```python
from build123d import *

# Parameters (mm, degrees)
F0_W     = 72.736366
F0_H     = 121.693536
F1_DEPTH = 19.05
F2_W     = 63.592366
F2_H     = 56.449744
F2_R     = 3.556
F2_W_2   = 5.08
F2_H_2   = 1.524
F3_DEPTH = 1.27
F4_R     = 5.08


with BuildPart() as f1:
    # F0 (on Front) → F1 (new body)
    with BuildSketch(Plane.XZ):
        Rectangle(F0_W, F0_H)
    extrude(amount=F1_DEPTH)

    # F2 (on face) → F3 (join)
    with BuildSketch(Plane.XZ.offset(19.05)):
        with Locations((0, 27.541896)):
            Rectangle(F2_W, F2_H)
        Polygon((-14.500647, -17.314185), (-22.619766, -17.314185), (-22.619766, -26.204185), (-29.613647, -26.204185), (-29.613647, -34.332185), (-22.628647, -34.332185), (-22.628647, -43.222185), (-14.500647, -43.222185), (-14.500647, -34.332185), (-7.515647, -34.332185), (-7.515647, -26.204185), (-14.500647, -26.204185), align=None)
        with Locations((30.073691, -19.163234)):
            Circle(F2_R)
        with Locations((19.722743, -25.038093)):
            Circle(F2_R)
        with Locations((-5.588, -54.265258)):
            Rectangle(F2_W_2, F2_H_2)
        with Locations((5.588, -54.265258)):
            Rectangle(F2_W_2, F2_H_2)
    extrude(amount=F3_DEPTH)

    # F4
    f4_edges = [f1.edges().sort_by_distance(p)[0] for p in [
        (-36.368183, -9.525, 60.846768),
        (36.368183, -9.525, 60.846768),
        (36.368183, -9.525, -60.846768),
        (-36.368183, -9.525, -60.846768),
    ]]
    fillet(f4_edges, radius=F4_R)


solid = f1.part
```
The listing builds one solid part. Answer for the finished solid, in the listing's coordinates (mm). A direction names the side the tool comes from. Coordinates: 2 decimals unless noted, no trailing zeros. Loops run counter-clockwise (first coordinate to the right, second up) from the corner with the lowest first, then second, coordinate; pieces in that order, holes last. Notation, with made-up numbers: M 59,-3 L 113,-3 A34 cw 113,27 Z; hole C 6.25,-4.5 d1. An arc over 180 degrees is marked long. Answer as a JSON object with one key per item and string values. Group by question number.
Item 1: Section A-A (x = -25.5) is taken. Write down the section's boundary in (y, z), and give its area (3 significant figures).
Item 2: Section C-C (x = 11) is taken. Write down the section's boundary in (y, z).
Item 3: Which of the six approach directions +Z, -Z, +X, -X, +Y, -Y give full straight-line access (tool end or side, diameter ignored) to faces 1 (the face through (0, -9, 60.847)), 2 (the face through (33.359, -19.676, -20.525))?
Item 4: Section B-B (z = -8.5) is taken. Write down the section's boundary in (x, y).
Item 5: Consider L1, parallel to Y at x = -19.5, z = -47.5; L2, parallel to X at y = -19.5, z = -36; L3, parallel to Z at x = 33, y = -1. Determine where each line is inside the solid, lowest interval first.
Item 6: Section D-D (x = 21.5) is taken. Write down the section's boundary in (y, z), and give its area (3 significant figures).
Item 7: Determine the mould class of faces 3 (the face through (0, -9, -60.847)), 4 (the face through (-1, -19.05, -13)), 5 (the face through (23.008, -19.676, -26.4)), 6 (the face through (0, -20.32, 28)) for opening direction Z: +Z half, -Z half, draft (parallel to the pull), parting line (faces both ways), or undercut.
Item 8: Each of these flat-tipped pins is pushed along its axis until it touches: P1, Ø0.6, axis at y = -20, z = -21.5, coming from the +X side; P2, Ø0.6, axis at y = -19.5, z = -38, coming from the -X side; P3, Ø1.4, axis at x = -3, y = -20, coming from the +Z side. Where does it stop, or does it pass through?
Solved:
{
 "1": {"outline": "M -20.32,-34.33 L -19.05,-34.33 L -19.05,-60.85 L 0,-60.85 L 0,60.85 L -19.05,60.85 L -19.05,55.77 L -20.32,55.77 L -20.32,-0.68 L -19.05,-0.68 L -19.05,-26.2 L -20.32,-26.2 Z", "area": "2,400 mm2"},
 "2": {"outline": "M -20.32,-0.68 L -19.05,-0.68 L -19.05,-60.85 L 0,-60.85 L 0,60.85 L -19.05,60.85 L -19.05,55.77 L -20.32,55.77 Z"},
 "3": {"face 1": "+Z, +X, -X, +Y, -Y", "face 2": "-Y"},
 "4": {"outline": "M -36.37,-19.05 L 36.37,-19.05 L 36.37,0 L -36.37,0 Z"},
 "5": {"L1": "y = -19.05 to 0", "L2": "x = -22.63 to -14.5", "L3": "z = -60.55 to 60.55"},
 "6": {"outline": "M -20.32,-28.12 L -19.05,-28.12 L -19.05,-60.85 L 0,-60.85 L 0,60.85 L -19.05,60.85 L -19.05,55.77 L -20.32,55.77 L -20.32,-0.68 L -19.05,-0.68 L -19.05,-21.96 L -20.32,-21.96 Z", "area": "2,400 mm2"},
 "7": {"face 3": "-Z half", "face 4": "undercut", "face 5": "undercut", "face 6": "draft"},
 "8": {"P1": "stops at x = 32.99", "P2": "stops at x = -22.63", "P3": "stops at z = 55.77"}
}
